from build123d import *

# Parameters (mm, degrees)
SKETCH1_R                  = 100
BOSS_EXTRUDE1_DEPTH        = 20
SKETCH2_R                  = 55
BOSS_EXTRUDE2_DEPTH        = 255
SKETCH3_R                  = 110
BOSS_EXTRUDE3_DEPTH        = 72.5
BOSS_EXTRUDE4_DEPTH        = 10
MIRROR4_COPY_1_DEPTH       = 10
MIRROR4_COPY_2_DEPTH       = 10
SKETCH5_R                  = 21
BOSS_EXTRUDE5_DEPTH        = 92
SKETCH7_R                  = 24
BOSS_EXTRUDE6_DEPTH        = 22
CUT_EXTRUDE1_DEPTH         = 5
SKETCH8_W                  = 278.540557596
SKETCH8_H                  = 4
BOSS_EXTRUDE7_DEPTH        = 15
F_13_0_13_DIAMETER_HOLE1_D = 13


with BuildPart() as part:
    # Sketch1 → Boss-Extrude1 (new body)
    with BuildSketch(Plane.XY):
        Circle(SKETCH1_R)
    extrude(amount=BOSS_EXTRUDE1_DEPTH)

    # Sketch2 → Boss-Extrude2 (add)
    with BuildSketch(Plane(origin=(0, 0, 0), x_dir=(-1, 0, 0), z_dir=(0, 0, -1))):
        Circle(SKETCH2_R)
    extrude(amount=BOSS_EXTRUDE2_DEPTH)

    # Sketch3 → Boss-Extrude3 (add, symmetric)
    with BuildSketch(Plane(origin=(0, 0, 0), x_dir=(0, 0, -1), z_dir=(1, 0, 0))):
        with Locations((137.5, -110)):
            Circle(SKETCH3_R)
    extrude(amount=BOSS_EXTRUDE3_DEPTH, both=True)

    # Sketch4 → Boss-Extrude4 (add)
    with BuildSketch(Plane(origin=(72.5, 0, 0), x_dir=(0, 0, -1), z_dir=(1, 0, 0))):
        with BuildLine():
            Line((-2.47558672, -280), (137.5, -280))
            Line((137.5, -280), (137.5, -200))
            ThreePointArc((137.5, -200), (73.860389693, -173.639610307), (47.5, -110))
            Line((47.5, -110), (27.5, -110))
            Line((27.5, -110), (-2.47558672, -280))
        make_face()
    boss_extrude4 = extrude(amount=BOSS_EXTRUDE4_DEPTH)

    # Mirror1: Boss-Extrude4 across plane
    add(boss_extrude4.mirror(Plane(origin=(82.5, 0, -137.5), x_dir=(1, 0, 0), z_dir=(0, 0, 1))))

    # Mirror3: Boss-Extrude4 across plane
    add(boss_extrude4.mirror(Plane(origin=(0, 0, 0), x_dir=(0, 0, 1), z_dir=(1, 0, 0))))

    # Mirror4 copy 1 sketch → Mirror4 copy 1 (add)
    with BuildSketch(Plane(origin=(-72.5, 0, -275), x_dir=(0, 0, 1), z_dir=(-1, 0, 0))):
        with BuildLine():
            Line((-2.47558672, -280), (137.5, -280))
            Line((137.5, -280), (137.5, -200))
            ThreePointArc((137.5, -200), (73.860389693, -173.639610307), (47.5, -110))
            Line((47.5, -110), (27.5, -110))
            Line((27.5, -110), (-2.47558672, -280))
        make_face()
    extrude(amount=MIRROR4_COPY_1_DEPTH)

    # Mirror4 copy 2 sketch → Mirror4 copy 2 (add)
    with BuildSketch(Plane(origin=(72.5, 0, -275), x_dir=(0, 0, 1), z_dir=(1, 0, 0))):
        with BuildLine():
            Line((-2.47558672, 280), (137.5, 280))
            Line((137.5, 280), (137.5, 200))
            ThreePointArc((137.5, 200), (73.860389693, 173.639610307), (47.5, 110))
            Line((47.5, 110), (27.5, 110))
            Line((27.5, 110), (-2.47558672, 280))
        make_face()
    extrude(amount=MIRROR4_COPY_2_DEPTH)

    # Sketch5 → Boss-Extrude5 (add)
    with BuildSketch(Plane(origin=(72.5, 0, 0), x_dir=(0, 0, -1), z_dir=(1, 0, 0))):
        with Locations((137.5, -110)):
            Circle(SKETCH5_R)
    extrude(amount=BOSS_EXTRUDE5_DEPTH)

    # Sketch7 → Boss-Extrude6 (add)
    with BuildSketch(Plane(origin=(72.5, 0, 0), x_dir=(0, 0, -1), z_dir=(1, 0, 0))):
        with Locations((137.5, -110)):
            Circle(SKETCH7_R)
    extrude(amount=BOSS_EXTRUDE6_DEPTH)

    # Sketch6 → Cut-Extrude1 (cut)
    with BuildSketch(Plane(origin=(0, -89, 0), x_dir=(1, 0, 0), z_dir=(0, 1, 0))):
        with BuildLine():
            Line((105.5, 143.5), (129.5, 143.5))
            Line((129.5, 143.5), (129.5, 131.5))
            Line((129.5, 131.5), (105.5, 131.5))
            ThreePointArc((105.5, 131.5), (99.5, 137.5), (105.5, 143.5))
        make_face()
    cut_extrude1 = extrude(amount=-CUT_EXTRUDE1_DEPTH, mode=Mode.SUBTRACT)

    # Mirror5: Cut-Extrude1 across plane
    add(cut_extrude1.mirror(Plane(origin=(129.5, -94, -143.5), x_dir=(0, 0, 1), z_dir=(1, 0, 0))), mode=Mode.SUBTRACT)

    # Sketch8 → Boss-Extrude7 (add)
    with BuildSketch(Plane(origin=(82.5, 0, 0), x_dir=(0, 0, -1), z_dir=(1, 0, 0))):
        with Locations((137.5, -278)):
            Rectangle(SKETCH8_W, SKETCH8_H)
    boss_extrude7 = extrude(amount=BOSS_EXTRUDE7_DEPTH)

    # Ø13.0 (13) Diameter Hole1 (through all)
    with Locations(Plane(origin=(0, -280, 0), x_dir=(-1, 0, 0), z_dir=(0, -1, 0))):
        with Locations((-90, 37.5), (-90, 237.5)):
            f_13_0_13_diameter_hole1 = Hole(F_13_0_13_DIAMETER_HOLE1_D / 2)

    # Mirror8: Boss-Extrude7, Ø13.0 (13) Diameter Hole1 across plane
    add(boss_extrude7.mirror(Plane(origin=(0, 0, 0), x_dir=(0, 0, 1), z_dir=(1, 0, 0))))
    add(f_13_0_13_diameter_hole1.mirror(Plane(origin=(0, 0, 0), x_dir=(0, 0, 1), z_dir=(1, 0, 0))), mode=Mode.SUBTRACT)


solid = part.part
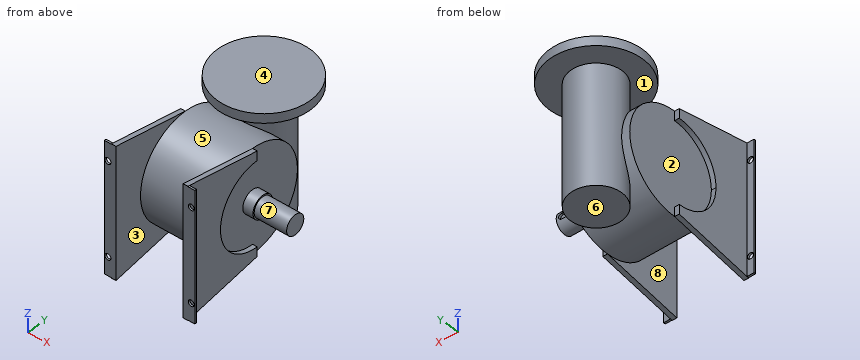
Work out the finished part from the listing and answer in its coordinate system (mm). Face numbers are marked on the shaded views. A direction names the side the tool comes from. Round coordinates to 2 decimals unless told otherwise and drop trailing zeros. Order: outer loops, then holes, each group sorted by start corner. A loop starts at its lowest first (then second) coordinate and runs counter-clockwise, first axis right, second up. Notation, with made-up numbers: M 16.5,89.25 L 30.5,89.25 A31 cw 30.5,113.25 Z; hole C -29.5,-3.5 d5. An arc over 180 degrees is marked long. Put each result on its own line as item: value. Start each with the question number.
Q1. Section B-B, the plane y = -69.5 is taken. Write down the section's boundary in (x, z).
Q2. Section A-A, the plane x = -90 is taken. Write down the section's boundary in (y, z), and give its area (3 significant figures).
Q3. A tool of negligible diameter and unlimited length cuts with its end or side. For the marked faces 4, 5, 6, 7 and 8, from which of +Z, -Z, +X, -X, +Y, -Y can it reach the whole face along a straight path? Write none if from no direction.
Q4. For a pull along X with two mould halves and no side action, classify the marked faces 1, 2 and 3 as pulls with the +X half, pulls with the -X half, needs draft (parallel to the pull), parting line crosses it, or undercut.
Q5. Flat-ended cylindrical pins translate along their axes: pin 1 (3 mm diameter, centred on x = 93, y = -278.5, fed in from -Z); pin 2 (4 mm diameter, centred on y = -41.5, z = -181.5, fed in from +X); pin 3 (4.5 mm diameter, centred on x = 122, y = -91.5, fed in from -Z); pin 4 (11.5 mm diameter, centred on x = -90, z = -37.5, fed in from -Y). Find the tip coordinate at first contact, or state that the pin passes through.
Q6. Section D-D, the plane x = 25.5 is taken. Write down the section's boundary in (y, z), and give its area (3 significant figures).
Q7. Section C-C, the plane z = -37.5 is taken. Write down the section's boundary in (x, y).
Q8. Straight lines are drawn through the part: L1, parallel to X at y = -278, z = -37; L2, parallel to Z at x = 90, y = -277; L3, parallel to X at y = -230.5, z = -54. For each, find the intervals that lie inside material, in ascending order. Write a range as [from, to].
Findings below:
1. outline: M -72.5,-239.77 L 72.5,-239.77 L 72.5,-35.23 L -72.5,-35.23 Z; M -71.9,0 L 71.9,0 L 71.9,20 L -71.9,20 Z
2. outline: M -280,-276.77 L -276,-276.77 L -276,-244 L -280,-244 Z; M -280,-231 L -276,-231 L -276,-44 L -280,-44 Z; M -280,-31 L -276,-31 L -276,1.77 L -280,1.77 Z; M -43.59,0 L 43.59,0 L 43.59,20 L -43.59,20 Z
2. area: 2,750 mm^2
3. face 4: +Z, +X, -X, +Y, -Y
3. face 5: none
3. face 6: -Z, +X, -X, +Y, -Y
3. face 7: +X
3. face 8: -Y
4. face 1: needs draft
4. face 2: pulls with the -X half
4. face 3: undercut
5. pin 1: stops at z = -276.77
5. pin 2: stops at x = 72.5
5. pin 3: stops at z = -150.8
5. pin 4: passes through
6. outline: M -96.69,0 L -48.73,0 L -48.73,-46.14 A110 ccw long -48.73,-228.86 L -48.73,-255 L 48.73,-255 L 48.73,0 L 96.69,0 L 96.69,20 L -96.69,20 Z
6. area: 60,500 mm^2
7. outline: M -97.5,-280 L -96.5,-280 L -96.5,-276 L -97.5,-276 Z; M -83.5,-280 L -72.5,-280 L -72.5,-155.83 L 72.5,-155.83 L 72.5,-280 L 83.5,-280 L 83.5,-276 L 82.5,-276 L 82.5,-110 L 72.5,-110 L 72.5,-64.17 L -72.5,-64.17 L -72.5,-110 L -82.5,-110 L -82.5,-276 L -83.5,-276 Z; C 0,0 d110; M 96.5,-280 L 97.5,-280 L 97.5,-276 L 96.5,-276 Z
8. L1: x = [-97.5, -96.48], [-83.52, -72.5], [72.5, 83.52], [96.48, 97.5]
8. L2: z = [-276.77, -244], [-231, -44], [-31, 1.77]
8. L3: x = [-82.5, -72.5], [72.5, 82.5]
